Verification items for this drawing (mm, ordinates from the low corner). Round coordinates to 2 decimals unless told otherwise and drop trailing zeros. Order: outer loops, then holes, each group sorted by start corner. A loop starts at its lowest first (then second) coordinate and runs counter-clockwise, first axis right, second up. Notation, with made-up numbers: (-11, 44) -> (0, 44) arc R23 ccw to (0, 61) -> close; hole circle Ø9 at (-32.75, -40). An arc over 180 degrees is marked (long way). Put each result on its own line as item: value.
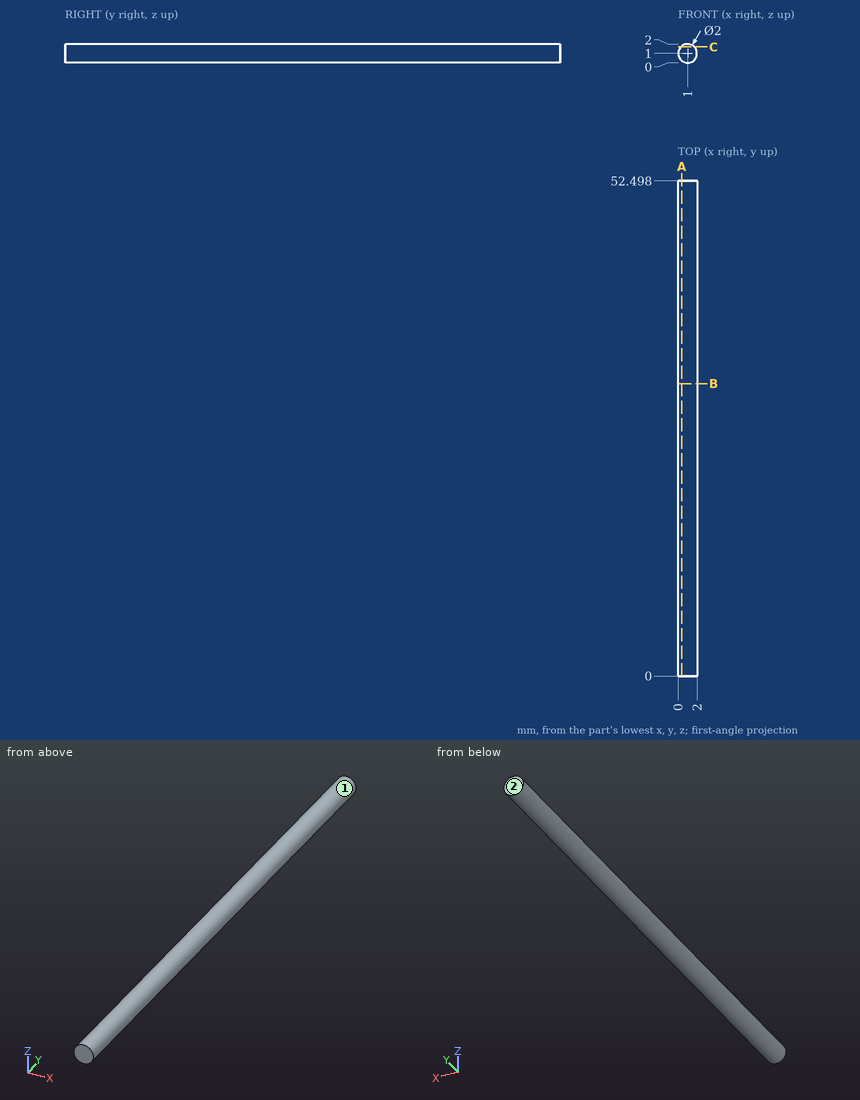
Item 1: Release check for a two-part mould opening along Z. For the marked faces 1 and 2 record: +Z half, -Z half, draft (parallel to the pull), parting line (faces both ways), or undercut.
Check sheet entries:
face 1: parting line
face 2: draft
Item 2: Material ranges on L1, parallel to X at y = 6, z = 1.1; L2, parallel to Z at x = 1.05, y = 32.5; L3, parallel to Z at x = 1.8, y = 24.5, recorded low to high. Write a range as [from, to].
Check sheet entries:
L1: x = [0.01, 1.99]
L2: z = [0, 2]
L3: z = [0.4, 1.6]
Item 3: Section check B-B on y = 31. Record the boundary of the cut face in (x, z).
Check sheet entries:
outline: circle Ø2 at (1, 1)
Item 4: Section check C-C on z = 1.7. Record the boundary of the cut face in (x, y), then the cut area to 3 significant figures.
Check sheet entries:
outline: (0.29, 0) -> (1.71, 0) -> (1.71, 52.5) -> (0.29, 52.5) -> close
area: 75.0 mm^2
Item 5: Section check A-A on x = 0.4. Record the boundary of the cut face in (y, z), then the cut area to 3 significant figures.
Check sheet entries:
outline: (0, 0.2) -> (52.5, 0.2) -> (52.5, 1.8) -> (0, 1.8) -> close
area: 84.0 mm^2
